Geometry: final body of the model. Coordinates: model frame, mm. A direction names the side the tool comes from. Give positions to 0.01 mm unless a question says otherwise; leave off trailing zeros. Order: outer loops, then holes, each group sorted by start corner. A loop starts at its lowest first (then second) coordinate and runs counter-clockwise, first axis right, second up. Notation, with made-up numbers: (42, 67) -> (64, 67) arc R25 cw to (64, 92) -> close; hole circle Ø5 at (-22.75, 29.25). An arc over 180 degrees is marked (long way). Write item = value, one per line.
```python
from build123d import *

# Parameters (mm, degrees)
SKETCH_1_W                      = 26
SKETCH_1_H                      = 33
EXTRUDE_1_DEPTH                 = 37
SKETCH_3_W                      = 26
SKETCH_3_H                      = 32
CUT_EXTRUDE_1_DEPTH             = 30
CUT_EXTRUDE_2_REACH             = 57.982
SKETCH_2_R                      = 0.75
CUT_EXTRUDE_2_DIRECTION_2_DEPTH = 56.982140009
CUT_EXTRUDE_3_REACH             = 57.982
SKETCH_4_R                      = 0.75
SKETCH_5_W                      = 17
SKETCH_5_H                      = 1.5
CUT_EXTRUDE_4_DEPTH             = 27
CUT_EXTRUDE_5_REACH             = 57.982
SKETCH_6_W                      = 20
SKETCH_6_H                      = 8
CUT_EXTRUDE_START               = -37
CUT_EXTRUDE_6_OUTLINE_R         = 0.75
CUT_EXTRUDE_6_DEPTH             = 37
SKETCH_8_W                      = 15
SKETCH_8_H                      = 1.5
CUT_EXTRUDE_7_DEPTH             = 13
SKETCH_9_R                      = 11
SKETCH_9_R_2                    = 10
EXTRUDE_2_DEPTH                 = 4
SKETCH_12_R                     = 10
EXTRUDE_3_DEPTH                 = 1.5
CUT_EXTRUDE_8_DEPTH             = 56.982140009
CUT_EXTRUDE_8_DEPTH_BACK        = 56.982140009
SKETCH_10_R                     = 1.8
SKETCH_11_R                     = 2.8
CUT_EXTRUDE_9_DEPTH             = 2.5


# Read off the part's stored shape, not the designer's step: 切除-拉伸6
with BuildPart() as part:
    # 草图1 → 凸台-拉伸1 (new body)
    with BuildSketch(Plane.XY):
        with Locations((13, 16.5)):
            Rectangle(SKETCH_1_W, SKETCH_1_H)
    extrude(amount=EXTRUDE_1_DEPTH)

    # 草图3 → 切除-拉伸1 (cut)
    with BuildSketch(Plane.XZ):
        with Locations((13, 18.5)):
            Rectangle(SKETCH_3_W, SKETCH_3_H)
    extrude(amount=-CUT_EXTRUDE_1_DEPTH, mode=Mode.SUBTRACT)

    # 草图2 → 切除-拉伸2 (cut, up to next)
    with BuildSketch(Plane.XY.offset(37), mode=Mode.PRIVATE) as cut_extrude_2_sk1:
        with Locations(Location((2.75, 1.5, 0), (0, 0, 180))):
            Circle(SKETCH_2_R)
    cut_extrude_2_tool1 = extrude(cut_extrude_2_sk1.sketch, amount=-CUT_EXTRUDE_2_REACH, mode=Mode.PRIVATE) & part.part
    # 草图2 → 切除-拉伸2 (cut, up to next)
    with BuildSketch(Plane.XY.offset(37), mode=Mode.PRIVATE) as cut_extrude_2_sk2:
        with Locations(Location((23.25, 1.5, 0), (0, 0, 180))):
            Circle(SKETCH_2_R)
    cut_extrude_2_tool2 = extrude(cut_extrude_2_sk2.sketch, amount=-CUT_EXTRUDE_2_REACH, mode=Mode.PRIVATE) & part.part
    # 草图2 → 切除-拉伸2 (cut, up to next)
    with BuildSketch(Plane.XY.offset(37), mode=Mode.PRIVATE) as cut_extrude_2_sk3:
        with Locations(Location((23.25, 22.2, 0), (0, 0, 180))):
            Circle(SKETCH_2_R)
    cut_extrude_2_tool3 = extrude(cut_extrude_2_sk3.sketch, amount=-CUT_EXTRUDE_2_REACH, mode=Mode.PRIVATE) & part.part
    # 草图2 → 切除-拉伸2 (cut, up to next)
    with BuildSketch(Plane.XY.offset(37), mode=Mode.PRIVATE) as cut_extrude_2_sk4:
        with Locations(Location((2.75, 22.2, 0), (0, 0, 180))):
            Circle(SKETCH_2_R)
    cut_extrude_2_tool4 = extrude(cut_extrude_2_sk4.sketch, amount=-CUT_EXTRUDE_2_REACH, mode=Mode.PRIVATE) & part.part
    add(cut_extrude_2_tool1.solids().sort_by_distance((2.75, 1.5, 37))[0], mode=Mode.SUBTRACT)
    add(cut_extrude_2_tool2.solids().sort_by_distance((23.25, 1.5, 37))[0], mode=Mode.SUBTRACT)
    add(cut_extrude_2_tool3.solids().sort_by_distance((23.25, 22.2, 37))[0], mode=Mode.SUBTRACT)
    add(cut_extrude_2_tool4.solids().sort_by_distance((2.75, 22.2, 37))[0], mode=Mode.SUBTRACT)

    # 草图2 → 切除-拉伸2 direction 2 (cut)
    with BuildSketch(Plane.XY.offset(37)):
        with Locations(Location((2.75, 1.5, 0), (0, 0, 180))):
            Circle(SKETCH_2_R)
        with Locations(Location((23.25, 1.5, 0), (0, 0, 180))):
            Circle(SKETCH_2_R)
        with Locations(Location((23.25, 22.2, 0), (0, 0, 180))):
            Circle(SKETCH_2_R)
        with Locations(Location((2.75, 22.2, 0), (0, 0, 180))):
            Circle(SKETCH_2_R)
    extrude(amount=CUT_EXTRUDE_2_DIRECTION_2_DEPTH, mode=Mode.SUBTRACT)

    # 草图4 → 切除-拉伸3 (cut, up to next)
    with BuildSketch(Plane(origin=(0, 0, 0), x_dir=(-1, 0, 0), z_dir=(0, 0, -1)), mode=Mode.PRIVATE) as cut_extrude_3_sk1:
        with Locations((-2.75, 1.5)):
            Circle(SKETCH_4_R)
    cut_extrude_3_tool1 = extrude(cut_extrude_3_sk1.sketch, amount=-CUT_EXTRUDE_3_REACH, mode=Mode.PRIVATE) & part.part
    # 草图4 → 切除-拉伸3 (cut, up to next)
    with BuildSketch(Plane(origin=(0, 0, 0), x_dir=(-1, 0, 0), z_dir=(0, 0, -1)), mode=Mode.PRIVATE) as cut_extrude_3_sk2:
        with Locations((-23.25, 1.5)):
            Circle(SKETCH_4_R)
    cut_extrude_3_tool2 = extrude(cut_extrude_3_sk2.sketch, amount=-CUT_EXTRUDE_3_REACH, mode=Mode.PRIVATE) & part.part
    # 草图4 → 切除-拉伸3 (cut, up to next)
    with BuildSketch(Plane(origin=(0, 0, 0), x_dir=(-1, 0, 0), z_dir=(0, 0, -1)), mode=Mode.PRIVATE) as cut_extrude_3_sk3:
        with Locations((-23.25, 25.95)):
            Circle(SKETCH_4_R)
    cut_extrude_3_tool3 = extrude(cut_extrude_3_sk3.sketch, amount=-CUT_EXTRUDE_3_REACH, mode=Mode.PRIVATE) & part.part
    # 草图4 → 切除-拉伸3 (cut, up to next)
    with BuildSketch(Plane(origin=(0, 0, 0), x_dir=(-1, 0, 0), z_dir=(0, 0, -1)), mode=Mode.PRIVATE) as cut_extrude_3_sk4:
        with Locations((-3.25, 25.95)):
            Circle(SKETCH_4_R)
    cut_extrude_3_tool4 = extrude(cut_extrude_3_sk4.sketch, amount=-CUT_EXTRUDE_3_REACH, mode=Mode.PRIVATE) & part.part
    add(cut_extrude_3_tool1.solids().sort_by_distance((2.75, 1.5, 0))[0], mode=Mode.SUBTRACT)
    add(cut_extrude_3_tool2.solids().sort_by_distance((23.25, 1.5, 0))[0], mode=Mode.SUBTRACT)
    add(cut_extrude_3_tool3.solids().sort_by_distance((23.25, 25.95, 0))[0], mode=Mode.SUBTRACT)
    add(cut_extrude_3_tool4.solids().sort_by_distance((3.25, 25.95, 0))[0], mode=Mode.SUBTRACT)

    # 草图5 → 切除-拉伸4 (cut)
    with BuildSketch(Plane.XZ):
        with Locations((13, 35.25)):
            Rectangle(SKETCH_5_W, SKETCH_5_H)
    extrude(amount=-CUT_EXTRUDE_4_DEPTH, mode=Mode.SUBTRACT)

    # 草图6 → 切除-拉伸5 (cut, up to next)
    with BuildSketch(Plane(origin=(0, 0, 0), x_dir=(-1, 0, 0), z_dir=(0, 0, -1)), mode=Mode.PRIVATE) as cut_extrude_5_sk1:
        with Locations((-13, 9)):
            Rectangle(SKETCH_6_W, SKETCH_6_H)
    cut_extrude_5_tool1 = extrude(cut_extrude_5_sk1.sketch, amount=-CUT_EXTRUDE_5_REACH, mode=Mode.PRIVATE) & part.part
    add(cut_extrude_5_tool1.solids().sort_by_distance((13, 9, 0))[0], mode=Mode.SUBTRACT)

    # 切除-拉伸6 outline → 切除-拉伸6 (cut)
    with BuildSketch(Plane(origin=(0, 0, 0), x_dir=(-1, 0, 0), z_dir=(0, 0, -1)).offset(CUT_EXTRUDE_START)):
        with BuildLine():
            Line((0, 0), (0, 13))
            Line((0, 13), (-13, 13))
            Line((-13, 13), (-13, 4))
            ThreePointArc((-13, 4), (-17.582575695, 2.947221814), (-21.246211251, 0))
            Line((-21.246211251, 0), (0, 0))
        make_face()
        with Locations((-2.75, 1.5)):
            Circle(CUT_EXTRUDE_6_OUTLINE_R, mode=Mode.SUBTRACT)
    extrude(amount=CUT_EXTRUDE_6_DEPTH, mode=Mode.SUBTRACT)

    # 草图8 → 切除-拉伸7 (cut)
    with BuildSketch(Plane.XZ.offset(-13)):
        with Locations((12.397702636, 1.75)):
            Rectangle(SKETCH_8_W, SKETCH_8_H)
    extrude(amount=-CUT_EXTRUDE_7_DEPTH, mode=Mode.SUBTRACT)

    # 草图9 → 凸台-拉伸2 (add)
    with BuildSketch(Plane(origin=(0, 33, 0), x_dir=(1, 0, 0), z_dir=(0, 1, 0))):
        with Locations(Location((13, -22, 0), (0, 0, 90))):
            Circle(SKETCH_9_R)
        with Locations(Location((13, -22, 0), (0, 0, 270))):
            Circle(SKETCH_9_R_2, mode=Mode.SUBTRACT)
    extrude(amount=EXTRUDE_2_DEPTH)

    # 草图12 → 凸台-拉伸3 (add)
    with BuildSketch(Plane(origin=(0, 33, 0), x_dir=(1, 0, 0), z_dir=(0, 1, 0))):
        with Locations(Location((13, -22, 0), (0, 0, 270))):
            Circle(SKETCH_12_R)
    extrude(amount=EXTRUDE_3_DEPTH)

    # 草图10 → 切除-拉伸8 (cut, two sides: drawn at the far end of the back side and taken through both)
    with BuildSketch(Plane(origin=(0, 33, 0), x_dir=(1, 0, 0), z_dir=(0, 1, 0)).offset(-CUT_EXTRUDE_8_DEPTH_BACK)):
        with Locations(Location((13, -15, 0), (0, 0, 270))):
            Circle(SKETCH_10_R)
        with Locations(Location((20, -22, 0), (0, 0, 270))):
            Circle(SKETCH_10_R)
        with Locations(Location((13, -29, 0), (0, 0, 270))):
            Circle(SKETCH_10_R)
        with Locations(Location((6, -22, 0), (0, 0, 270))):
            Circle(SKETCH_10_R)
    extrude(amount=CUT_EXTRUDE_8_DEPTH + CUT_EXTRUDE_8_DEPTH_BACK, mode=Mode.SUBTRACT)

    # 草图11 → 切除-拉伸9 (cut)
    with BuildSketch(Plane.XZ.offset(-30)):
        with Locations(Location((6, 22, 0), (0, 0, 270))):
            Circle(SKETCH_11_R)
        with Locations(Location((13, 29, 0), (0, 0, 270))):
            Circle(SKETCH_11_R)
        with Locations(Location((20, 22, 0), (0, 0, 270))):
            Circle(SKETCH_11_R)
        with Locations(Location((13, 15, 0), (0, 0, 270))):
            Circle(SKETCH_11_R)
    extrude(amount=-CUT_EXTRUDE_9_DEPTH, mode=Mode.SUBTRACT)


solid = part.part
```
1) Section query C-C (z = 29). Output: boundary loops of the cut face in (x, y).
Check sheet entries:
outline = (0, 30) -> (10.2, 30) -> (10.2, 32.5) -> (11.2, 32.5) -> (11.2, 34.5) -> (5.86, 34.5) -> (5.86, 37) -> (4.51, 37) -> (4.51, 33) -> (0, 33) -> close; (14.8, 32.5) -> (15.8, 32.5) -> (15.8, 30) -> (26, 30) -> (26, 33) -> (21.49, 33) -> (21.49, 37) -> (20.14, 37) -> (20.14, 34.5) -> (14.8, 34.5) -> close
2) Reachability of faces 5 (the face through (21, 18, 2.5)), 6 (the face through (16, 35.73, 31.54)), 7 (the face through (18, 5, 1)), 8 (the face through (24, 26, 1)), 9 (the face through (4.296, 31.232, 24.222)) from +Z, -Z, +X, -X, +Y, -Y: full face, straight path, thin tool, end or side. Return the list, or none.
Check sheet entries:
face_5 = +X, -X, -Y
face_6 = +Y
face_7 = -Z, -X
face_8 = -Z
face_9 = -Y
3) Section query B-B (y = 22.2). Output: boundary loops of the cut face in (x, z), plus the area to 3 significant figures.
Check sheet entries:
outline = (0, 0) -> (26, 0) -> (26, 2.5) -> (19.9, 2.5) -> (19.9, 1) -> (4.9, 1) -> (4.9, 2.5) -> (0, 2.5) -> close; (0, 34.5) -> (2, 34.5) -> (2, 37) -> (0, 37) -> close; (3.5, 34.5) -> (4.5, 34.5) -> (4.5, 36) -> (21.5, 36) -> (21.5, 34.5) -> (22.5, 34.5) -> (22.5, 37) -> (3.5, 37) -> close; (24, 34.5) -> (26, 34.5) -> (26, 37) -> (24, 37) -> close
area = 74.5 mm²
4) Mould query, pull axis Z, two halves, no side actions, for faces 1 (the face through (11, 32.5, 15)), 2 (the face through (4.403, 33.486, 22.831)), 3 (the face through (13, 20, 37)), 4 (the face through (0, 30.4, 18.4)). Classes: +Z half, -Z half, draft (parallel to the pull), parting line (faces both ways), or undercut.
Check sheet entries:
face_1 = undercut
face_2 = undercut
face_3 = +Z half
face_4 = draft
5) Section query D-D (z = 3.5). Output: boundary loops of the cut face in (x, y), plus the area to 3 significant figures.
Check sheet entries:
outline = (0, 30) -> (26, 30) -> (26, 33) -> (0, 33) -> close
area = 78.0 mm²
6) Line query: line 1 (Y direction, x = 23.25, z = 0.5); line 2 (Z direction, x = 5, y = 20.5); line 3 (Z direction, x = 1.5, y = 16). Output: solid intervals per line, ascending. Write a range as from..to.
Check sheet entries:
line_1 = 0..0.75, 2.25..25.2, 26.7..33
line_2 = 0..1, 36..37
line_3 = 0..2.5, 34.5..37
7) First-contact query: P1, Ø4.5, axis at x = 20.5, z = 21.5, coming from the -Y side; P2, Ø4, axis at y = 26, z = 32, coming from the -X side; P3, Ø0.8, axis at x = 16.5, z = 1, coming from the -Y side; P4, Ø2, axis at x = 10, z = 20, coming from the +Y side. Flat tips, straight axial feed; report the tip coordinate or a pass-through.
Check sheet entries:
P1 = 30
P2 = through
P3 = 3.25
P4 = 34.5
8) Section query A-A (y = 8.5). Output: boundary loops of the cut face in (x, z), plus the area to 4 significant figures.
Check sheet entries:
outline = (13, 36) -> (21.5, 36) -> (21.5, 34.5) -> (26, 34.5) -> (26, 37) -> (13, 37) -> close; (23, 0) -> (26, 0) -> (26, 2.5) -> (23, 2.5) -> close
area = 27.25 mm²
